Verification items for the finished model (mm, model axes). A direction names the side the tool comes from. Coordinates: 2 decimals unless noted, no trailing zeros. Loops run counter-clockwise (first coordinate to the right, second up) from the corner with the lowest first, then second, coordinate; pieces in that order, holes last. Notation, with made-up numbers: (80, -31.75) -> (116, -31.75) arc R28 ccw to (116, -10.75) -> close; hole circle Ø10 at (64, -24.75). An arc over 180 degrees is marked (long way). Answer as a JSON object with one key per item and string values. Group by question number.
Q1. Scan lines: L1, parallel to X at y = 12, z = 8.5; L2, parallel to Y at x = 4.75, z = 1; L3, parallel to Y at x = -9.5, z = 9.25. Record each from-to range of solid material in increasing order.
Q2. Set-up check for faces 1 (the cylindrical face through (-10.15, 34.68, 5.07)), 2 (the flat face through (12.35, 0, 5)): record each of +Z, -Z, +X, -X, +Y, -Y from which the full face is reachable in a straight line by a thin tool's end or side.
Q3. Cross-section at C-C on y = 6.5. Record the boundary of the cut face in (x, z), and give its area (3 significant figures).
Q4. Cross-section at A-A on x = 7.25. Record the boundary of the cut face in (y, z).
Q5. Cross-section at B-B on z = 1.75. Record the boundary of the cut face in (x, y), and give its area (3 significant figures).
Q6. Release check for a two-part mould opening along X. For faces 3 (the flat face through (10.75, 0, 5)), 4 (the cylindrical face through (10.15, -34.68, 5.07)), 5 (the flat face through (0, 36.85, 5)), 6 (the cylindrical face through (-11.75, 36.28, 5.07)) record: released by +X, released by -X, zero draft, split by the parting line, or undercut.
Autodesk Inventor part; units mm, degrees
ref_plane "YZ Plane" through (0, 0, 0) normal (1, 0, 0) x (0, 1, 0)
ref_plane "XZ Plane" through (0, 0, 0) normal (0, 1, 0) x (-1, 0, 0)
ref_plane "XY Plane" through (0, 0, 0) normal (0, 0, 1) x (1, 0, 0)
sketch "Sketch1" plane through (0, 0, 0) normal (0, 0, 1) x (1, 0, 0)
  line L0 (-10.75, 35.25) -> (10.75, 35.25)
  line L1 (10.75, 35.25) -> (10.75, -35.25)
  line L2 (10.75, -35.25) -> (-10.75, -35.25)
  line L3 (-10.75, -35.25) -> (-10.75, 35.25)
  line L4 (12.35, 36.85) -> (-12.35, 36.85)
  line L5 (-12.35, 36.85) -> (-12.35, -36.85)
  line L6 (-12.35, -36.85) -> (12.35, -36.85)
  line L7 (12.35, -36.85) -> (12.35, 36.85)
  point P0 (0, 0)
  point P1 (10.75, 0)
  point P2 (0, 35.25)
  dimension "d0" = 21.5
  dimension "d1" = 70.5
  dimension "d2" = 1.6
extrude "Extrusion1" add sketch "Sketch1" along normal blind 10
fillet "Fillet1" radius 2 7 edges at (12.35, 36.85, 5) (10.75, 35.25, 5) (-10.75, 35.25, 5) (-12.35, 36.85, 5) (-12.35, -36.85, 5) (12.35, -36.85, 5) (10.75, -35.25, 5)
properties part number "SampleHolderBand" material "ABS Plastic"
Computed values:
{
 "1": {"L1": "x = -12.35 to -10.75, 10.75 to 12.35", "L2": "y = -36.85 to -35.25, 35.25 to 36.85", "L3": "y = -36.85 to -35.25, 35.1 to 36.85"},
 "2": {"face 1": "+Z, -Z", "face 2": "+Z, -Z, +X, +Y, -Y"},
 "3": {"outline": "(-12.35, 0) -> (-10.75, 0) -> (-10.75, 10) -> (-12.35, 10) -> close; (10.75, 0) -> (12.35, 0) -> (12.35, 10) -> (10.75, 10) -> close", "area": "32.0 mm²"},
 "4": {"outline": "(-36.85, 0) -> (-35.25, 0) -> (-35.25, 10) -> (-36.85, 10) -> close; (35.25, 0) -> (36.85, 0) -> (36.85, 10) -> (35.25, 10) -> close"},
 "5": {"outline": "(-12.35, -34.85) arc R2 ccw to (-10.35, -36.85) -> (10.35, -36.85) arc R2 ccw to (12.35, -34.85) -> (12.35, 34.85) arc R2 ccw to (10.35, 36.85) -> (-10.35, 36.85) arc R2 ccw to (-12.35, 34.85) -> close; hole (-10.75, -35.25) -> (8.75, -35.25) arc R2 ccw to (10.75, -33.25) -> (10.75, 33.25) arc R2 ccw to (8.75, 35.25) -> (-8.75, 35.25) arc R2 ccw to (-10.75, 33.25) -> close", "area": "304 mm²"},
 "6": {"face 3": "undercut", "face 4": "undercut", "face 5": "zero draft", "face 6": "released by -X"}
}
